```python
from build123d import *

# Parameters (mm, degrees)
SKETCH1_W           = 132
SKETCH1_H           = 160
BOSS_EXTRUDE1_DEPTH = 6
SKETCH3_W           = 32
SKETCH3_H           = 54
SKETCH3_W_2         = 26
SKETCH3_H_2         = 48
BOSS_EXTRUDE2_DEPTH = 17.5
SKETCH4_W           = 32
SKETCH4_H           = 54
BOSS_EXTRUDE3_DEPTH = 3
SKETCH5_W           = 25
SKETCH5_H           = 17
CUT_EXTRUDE1_DEPTH  = 3
SKETCH6_W           = 12
SKETCH6_H           = 54
BOSS_EXTRUDE4_DEPTH = 3
SKETCH7_R           = 1.6
CUT_EXTRUDE2_DEPTH  = 106.177231376
SKETCH8_W           = 3
SKETCH8_H           = 6.5
BOSS_EXTRUDE5_DEPTH = 20
SKETCH9_R           = 1.55
CUT_EXTRUDE3_DEPTH  = 6
SKETCH10_R          = 1.6
CUT_EXTRUDE4_DEPTH  = 108.043215572
SKETCH11_W          = 2.5
SKETCH11_H          = 7
BOSS_EXTRUDE6_DEPTH = 19.36
SKETCH12_R          = 1.6
CUT_EXTRUDE5_DEPTH  = 19.36
SKETCH13_W          = 3
SKETCH13_H          = 7
BOSS_EXTRUDE7_DEPTH = 15
SKETCH14_R          = 2
CUT_EXTRUDE6_DEPTH  = 15
CUT_EXTRUDE7_START  = -6
CUT_EXTRUDE7_DEPTH  = 6
SKETCH16_R          = 1.6
CUT_EXTRUDE8_DEPTH  = 15
SKETCH17_W          = 119.064494472
SKETCH17_H          = 144.515611373
CUT_EXTRUDE10_DEPTH = 61


# Read off the part's stored shape, not the designer's step: Cut-Extrude7
with BuildPart() as part:
    # Sketch1 → Boss-Extrude1 (new body)
    with BuildSketch(Plane.XY):
        Rectangle(SKETCH1_W, SKETCH1_H)
    extrude(amount=BOSS_EXTRUDE1_DEPTH)

    # Sketch3 → Boss-Extrude2 (add)
    with BuildSketch(Plane.XY.offset(6)):
        with Locations((0, -53)):
            Rectangle(SKETCH3_W, SKETCH3_H)
        with Locations((0, -53)):
            Rectangle(SKETCH3_W_2, SKETCH3_H_2, mode=Mode.SUBTRACT)
    extrude(amount=BOSS_EXTRUDE2_DEPTH)

    # Sketch4 → Boss-Extrude3 (add)
    with BuildSketch(Plane.XY.offset(23.5)):
        with Locations((0, -53)):
            Rectangle(SKETCH4_W, SKETCH4_H)
    extrude(amount=BOSS_EXTRUDE3_DEPTH)

    # Sketch5 → Cut-Extrude1 (cut)
    with BuildSketch(Plane.XZ.offset(80)):
        with Locations((0, 14.5)):
            Rectangle(SKETCH5_W, SKETCH5_H)
    extrude(amount=-CUT_EXTRUDE1_DEPTH, mode=Mode.SUBTRACT)

    # Sketch6 → Boss-Extrude4 (add)
    with BuildSketch(Plane.XY.offset(6)):
        with Locations((-22, -53)):
            Rectangle(SKETCH6_W, SKETCH6_H)
        with Locations((22, -53)):
            Rectangle(SKETCH6_W, SKETCH6_H)
    extrude(amount=BOSS_EXTRUDE4_DEPTH)

    # Sketch7 → Cut-Extrude2 (cut, through all)
    with BuildSketch(Plane.XY.offset(9)):
        with Locations((-22, -69)):
            Circle(SKETCH7_R)
        with Locations((-22, -33)):
            Circle(SKETCH7_R)
        with Locations(Location((22, -69, 0), (0, 0, 180))):
            Circle(SKETCH7_R)
        with Locations(Location((22, -33, 0), (0, 0, 180))):
            Circle(SKETCH7_R)
    extrude(amount=-CUT_EXTRUDE2_DEPTH, mode=Mode.SUBTRACT)

    # Sketch8 → Boss-Extrude5 (add)
    with BuildSketch(Plane.XY.offset(6)):
        with Locations((-54.38, -76.75)):
            Rectangle(SKETCH8_W, SKETCH8_H)
        with Locations((-54.38, -30.25)):
            Rectangle(SKETCH8_W, SKETCH8_H)
    boss_extrude5 = extrude(amount=BOSS_EXTRUDE5_DEPTH)

    # Sketch9 → Cut-Extrude3 (cut)
    with BuildSketch(Plane.ZY.offset(55.88)):
        with Locations((10.35, -76.75)):
            Circle(SKETCH9_R)
        with Locations((19.65, -76.75)):
            Circle(SKETCH9_R)
        with Locations((10.35, -30.25)):
            Circle(SKETCH9_R)
        with Locations((19.65, -30.25)):
            Circle(SKETCH9_R)
    cut_extrude3 = extrude(amount=-CUT_EXTRUDE3_DEPTH, mode=Mode.SUBTRACT)

    # Mirror1: Boss-Extrude5, Cut-Extrude3 across plane
    add(boss_extrude5.mirror(Plane(origin=(0, 0, 0), x_dir=(0, 0, 1), z_dir=(1, 0, 0))))
    add(cut_extrude3.mirror(Plane(origin=(0, 0, 0), x_dir=(0, 0, 1), z_dir=(1, 0, 0))), mode=Mode.SUBTRACT)

    # Sketch10 → Cut-Extrude4 (cut, through all)
    with BuildSketch(Plane(origin=(0, 0, 0), x_dir=(-1, 0, 0), z_dir=(0, 0, -1))):
        with Locations((-24.1, -75.572749788)):
            Circle(SKETCH10_R)
        with Locations((-21.15, -12.732749788)):
            Circle(SKETCH10_R)
        with Locations(Location((21.15, -12.732749788, 0), (0, 0, 180))):
            Circle(SKETCH10_R)
        with Locations((24.1, -75.572749788)):
            Circle(SKETCH10_R)
    extrude(amount=-CUT_EXTRUDE4_DEPTH, mode=Mode.SUBTRACT)

    # Sketch11 → Boss-Extrude6 (add)
    with BuildSketch(Plane(origin=(0, 0, 0), x_dir=(-1, 0, 0), z_dir=(0, 0, -1))):
        with Locations((-17.9, 1.267250212)):
            Rectangle(SKETCH11_W, SKETCH11_H)
        with Locations((-17.9, 50.267250212)):
            Rectangle(SKETCH11_W, SKETCH11_H)
    extrude(amount=BOSS_EXTRUDE6_DEPTH)

    # Sketch12 → Cut-Extrude5 (cut)
    with BuildSketch(Plane(origin=(19.15, 0, 0), x_dir=(0, 0, -1), z_dir=(1, 0, 0))):
        with Locations(Location((4.5, 50.267250212, 0), (0, 0, 90))):
            Circle(SKETCH12_R)
        with Locations(Location((14.5, 50.267250212, 0), (0, 0, 90))):
            Circle(SKETCH12_R)
        with Locations(Location((4.5, 1.267250212, 0), (0, 0, 90))):
            Circle(SKETCH12_R)
        with Locations(Location((14.5, 1.267250212, 0), (0, 0, 90))):
            Circle(SKETCH12_R)
    extrude(amount=-CUT_EXTRUDE5_DEPTH, mode=Mode.SUBTRACT)

    # Sketch13 → Boss-Extrude7 (add)
    with BuildSketch(Plane(origin=(0, 0, 0), x_dir=(-1, 0, 0), z_dir=(0, 0, -1))):
        with Locations((29.35, 35.967250212)):
            Rectangle(SKETCH13_W, SKETCH13_H)
    extrude(amount=BOSS_EXTRUDE7_DEPTH)

    # Sketch14 → Cut-Extrude6 (cut)
    with BuildSketch(Plane.ZY.offset(30.85)):
        with Locations((-9.9, 35.967250212)):
            Circle(SKETCH14_R)
    extrude(amount=-CUT_EXTRUDE6_DEPTH, mode=Mode.SUBTRACT)

    # Cut-Extrude7 outline → Cut-Extrude7 (cut)
    with BuildSketch(Plane(origin=(0, 0, 0), x_dir=(-1, 0, 0), z_dir=(0, 0, -1)).offset(CUT_EXTRUDE7_START)):
        Polygon((-30.85, 56.767250212), (30.85, 56.767250212), (30.85, -24), (58.88, -24), (58.88, -80), (66, -80), (66, 80), (-66, 80), (-66, -80), (-58.88, -80), (-58.88, -24), (-30.85, -24), align=None)
    extrude(amount=CUT_EXTRUDE7_DEPTH, mode=Mode.SUBTRACT)

    # Sketch16 → Cut-Extrude8 (cut)
    with BuildSketch(Plane(origin=(0, 0, 0), x_dir=(-1, 0, 0), z_dir=(0, 0, -1))):
        Circle(SKETCH16_R)
        with Locations((0, 52.767250212)):
            Circle(SKETCH16_R)
    extrude(amount=-CUT_EXTRUDE8_DEPTH, mode=Mode.SUBTRACT)

    # Sketch17 → Cut-Extrude10 (cut)
    with BuildSketch(Plane.XY.offset(6)):
        with Locations((0.652247236, -7.742194314)):
            Rectangle(SKETCH17_W, SKETCH17_H)
    extrude(amount=-CUT_EXTRUDE10_DEPTH, mode=Mode.SUBTRACT)


with BuildPart() as body_2:
    # of the pieces the cut leaves, the one that is kept (cut_extrude10_keep)
    add(part.part.solids().sort_by_distance((12.5, -80, 6))[0])


solid = body_2.part
```
Design review of the part built by this model. Coordinates are the model's own, in mm. A direction names the side the tool comes from. Round coordinates to 2 decimals unless told otherwise and drop trailing zeros. Order: outer loops, then holes, each group sorted by start corner. A loop starts at its lowest first (then second) coordinate and runs counter-clockwise, first axis right, second up. Notation, with made-up numbers: (-26, -26) - (-3, -26) arc R12 ccw to (-3, -10) - close; hole circle Ø5 at (57, 73). An arc over 180 degrees is marked (long way). Return JSON: item names as keys, results as strings.
Q1. For pin 1 Ø2.5 at (x, y) = (-22, -33) entering from +Z; pin 2 Ø2 at (x, y) = (4.5, -66.5) entering from -Z; pin 3 Ø2 at (x, z) = (-7.5, 16.5) entering from -Y; pin 4 Ø1.5 at (x, y) = (-3.5, -79) entering from -Z, all flat-tipped, find the tip position at first contact; note any pin that passes through.
Computed values:
{"pin 1": "passes through", "pin 2": "stops at z = 23.5", "pin 3": "stops at y = -29", "pin 4": "stops at z = 23"}
Q2. The part is to be moulded in two halves that separate along Y. For faces 1 (the flat face through (0, -26, 16)), 2 (the cylindrical face through (23.24, -74.224, 7.479)), 3 (the flat face through (12.5, -79, 14)), say which applies: pulls with the +Y half, pulls with the -Y half, needs draft (parallel to the pull), parting line crosses it, or undercut.
Computed values:
{"face 1": "pulls with the +Y half", "face 2": "undercut", "face 3": "needs draft"}
Q3. Wall thickness on L1, parallel to X at y = -69, z = 8.25; L2, parallel to Y at x = -22, z = 7.95; L3, parallel to X at y = -60.5, z = 23.25: over which ranges is each line inside the solid? List them lowest first. Write a range as [from, to].
Computed values:
{"L1": "x = [-28, -23.6], [-20.4, -13], [13, 20.4], [23.6, 28]", "L2": "y = [-80, -70.6], [-67.4, -34.6], [-31.4, -26]", "L3": "x = [-16, -13], [13, 16]"}
Q4. Consider section C-C on z = 7.5. Write out the cut boundary in (x, y).
Computed values:
{"outline": "(-28, -80) - (-12.5, -80) - (-12.5, -77) - (-13, -77) - (-13, -29) - (13, -29) - (13, -77) - (12.5, -77) - (12.5, -80) - (28, -80) - (28, -26) - (-28, -26) - close; hole circle Ø3.2 at (-24.1, -75.57); hole circle Ø3.2 at (-22, -69); hole circle Ø3.2 at (-22, -33); hole circle Ø3.2 at (22, -69); hole circle Ø3.2 at (22, -33); hole circle Ø3.2 at (24.1, -75.57)"}
Q5. Consider section A-A on z = 18.75. Write out the cut boundary in (x, y), plus the area to 3 significant figures.
Computed values:
{"outline": "(-16, -80) - (-12.5, -80) - (-12.5, -77) - (-13, -77) - (-13, -29) - (13, -29) - (13, -77) - (12.5, -77) - (12.5, -80) - (16, -80) - (16, -26) - (-16, -26) - close", "area": "405 mm2"}
Q6. Machinability: for faces 4 (the flat face through (16, -53, 18)), 5 (the flat face through (-13, -53, 15)), 6 (the flat face through (-22, -53, 9)), which of the approach directions +Z, -Z, +X, -X, +Y, -Y give a long, thin tool a straight path to every point of the face, cutting with its end or side? Answer none if there is none.
Computed values:
{"face 4": "+Z, +X, +Y, -Y", "face 5": "-Z", "face 6": "+Z, -X, +Y, -Y"}
Q7. Consider section D-D on x = -3.5. Write out the cut boundary in (y, z).
Computed values:
{"outline": "(-80, 23) - (-77, 23) - (-77, 23.5) - (-29, 23.5) - (-29, 6) - (-26, 6) - (-26, 26.5) - (-80, 26.5) - close"}
Q8. Consider section B-B on y = -58. Write out the cut boundary in (x, z), plus the area to 3 significant figures.
Computed values:
{"outline": "(-28, 6) - (-13, 6) - (-13, 23.5) - (13, 23.5) - (13, 6) - (28, 6) - (28, 9) - (16, 9) - (16, 26.5) - (-16, 26.5) - (-16, 9) - (-28, 9) - close", "area": "273 mm2"}
